The listing builds one solid part. Answer for the finished solid, in the listing's coordinates (mm). A direction names the side the tool comes from. Coordinates: 2 decimals unless noted, no trailing zeros. Loops run counter-clockwise (first coordinate to the right, second up) from the corner with the lowest first, then second, coordinate; pieces in that order, holes last. Notation, with made-up numbers: (0, 2) -> (30, 2) arc R22 cw to (30, 11) -> close; hole circle Ø10 at (-6, -1.75). An arc over 180 degrees is marked (long way). Answer in a Markdown table with one row per item.
```python
from build123d import *

# Parameters (mm, degrees)
EXTRUDE_1_DEPTH          = 18
SKETCH_3_R               = 2.75
CUT_EXTRUDE_1_DEPTH      = 1
CUT_EXTRUDE_1_DEPTH_BACK = 41
CUT_EXTRUDE_2_REACH      = 42
SKETCH_4_R               = 2.75


with BuildPart() as part:
    # 草图1 → 凸台-拉伸1 (new body)
    with BuildSketch(Plane(origin=(0, 0, 0), x_dir=(0, 0, -1), z_dir=(1, 0, 0))):
        Polygon((0, 0), (0, -40), (40, -40), (40, -37), (3, -37), (3, 0), align=None)
    extrude(amount=EXTRUDE_1_DEPTH)

    # 草图3 → 切除-拉伸1 (cut, two sides)
    with BuildSketch(Plane.XZ.offset(40)) as cut_extrude_1_sk:
        with Locations((9, -10)):
            Circle(SKETCH_3_R)
        with Locations((9, -30)):
            Circle(SKETCH_3_R)
    extrude(amount=CUT_EXTRUDE_1_DEPTH, mode=Mode.SUBTRACT)
    extrude(cut_extrude_1_sk.sketch, amount=-CUT_EXTRUDE_1_DEPTH_BACK, mode=Mode.SUBTRACT)

    # 草图4 → 切除-拉伸2 (cut, up to next)
    with BuildSketch(Plane(origin=(0, 0, 0), x_dir=(-1, 0, 0), z_dir=(0, 0, 1)), mode=Mode.PRIVATE) as cut_extrude_2_sk1:
        with Locations((-9, 30)):
            Circle(SKETCH_4_R)
    cut_extrude_2_tool1 = extrude(cut_extrude_2_sk1.sketch, amount=-CUT_EXTRUDE_2_REACH, mode=Mode.PRIVATE) & part.part
    add(cut_extrude_2_tool1.solids().sort_by_distance((9, -30, 0))[0], mode=Mode.SUBTRACT)
    # 草图4 → 切除-拉伸2 (cut, up to next)
    with BuildSketch(Plane(origin=(0, 0, 0), x_dir=(-1, 0, 0), z_dir=(0, 0, 1)), mode=Mode.PRIVATE) as cut_extrude_2_sk2:
        with Locations((-9, 10)):
            Circle(SKETCH_4_R)
    cut_extrude_2_tool2 = extrude(cut_extrude_2_sk2.sketch, amount=-CUT_EXTRUDE_2_REACH, mode=Mode.PRIVATE) & part.part
    add(cut_extrude_2_tool2.solids().sort_by_distance((9, -10, 0))[0], mode=Mode.SUBTRACT)


solid = part.part
```
Item 1: A cutting plane is placed at C-C, the plane y = -30. Determine the outline of the cut face in (x, z).
Findings below:
| item | result |
|---|---|
| outline | (0, -3) -> (6.25, -3) -> (6.25, 0) -> (0, 0) -> close; (11.75, -3) -> (18, -3) -> (18, 0) -> (11.75, 0) -> close |
Item 2: A cutting plane is placed at D-D, the plane x = 12.5. Determine the outline of the cut face in (y, z), plus the area to 3 significant figures.
Findings below:
| item | result |
|---|---|
| outline | (-40, -40) -> (-37, -40) -> (-37, -3) -> (0, -3) -> (0, 0) -> (-40, 0) -> close |
| area | 231 mm2 |
Item 3: Find the intervals of material crossed by probe 1 along Y at (x, z) = (9, -0.8); probe 2 along X at (y, z) = (-10, -1), in increasing order.
Findings below:
| item | result |
|---|---|
| probe 1 | y = -40 to -32.75, -27.25 to -12.75, -7.25 to 0 |
| probe 2 | x = 0 to 6.25, 11.75 to 18 |
Item 4: Flat-ended cylindrical pins translate along their axes: pin 1 Ø4.5 at (x, y) = (9, -30) entering from +Z; pin 2 Ø1 at (x, y) = (2, -5) entering from -Z; pin 3 Ø8 at (x, z) = (2, -15.5) entering from +Y. Find the tip coordinate at first contact, or state that the pin passes through.
Findings below:
| item | result |
|---|---|
| pin 1 | passes through |
| pin 2 | stops at z = -3 |
| pin 3 | stops at y = -37 |
Item 5: A cutting plane is placed at A-A, the plane z = -30. Determine the outline of the cut face in (x, y), plus the area to 3 significant figures.
Findings below:
| item | result |
|---|---|
| outline | (0, -40) -> (6.25, -40) -> (6.25, -37) -> (0, -37) -> close; (11.75, -40) -> (18, -40) -> (18, -37) -> (11.75, -37) -> close |
| area | 37.5 mm2 |
Item 6: A tool of negligible diameter and unlimited length cuts with its end or side. For faces 1 (the face through (9, 0, -2)), 2 (the face through (9, -19, -3)), from which of +Z, -Z, +X, -X, +Y, -Y can it reach the whole face along a straight path? Write none if from no direction.
Findings below:
| item | result |
|---|---|
| face 1 | +Z, -Z, +X, -X, +Y |
| face 2 | -Z, +X, -X, +Y |
Item 7: Determine the mould class of faces 3 (the face through (9, -20, 0)), 4 (the face through (7.52, -32.32, -1.48)), 5 (the face through (9, -37, -22)), 6 (the face through (9, -40, -20)) for opening direction Y: +Y half, -Y half, draft (parallel to the pull), parting line (faces both ways), or undercut.
Findings below:
| item | result |
|---|---|
| face 3 | draft |
| face 4 | undercut |
| face 5 | +Y half |
| face 6 | -Y half |
Item 8: A cutting plane is placed at B-B, the plane x = 9. Determine the outline of the cut face in (y, z).
Findings below:
| item | result |
|---|---|
| outline | (-40, -40) -> (-37, -40) -> (-37, -32.75) -> (-40, -32.75) -> close; (-40, -27.25) -> (-37, -27.25) -> (-37, -12.75) -> (-40, -12.75) -> close; (-40, -7.25) -> (-37, -7.25) -> (-37, -3) -> (-32.75, -3) -> (-32.75, 0) -> (-40, 0) -> close; (-27.25, -3) -> (-12.75, -3) -> (-12.75, 0) -> (-27.25, 0) -> close; (-7.25, -3) -> (0, -3) -> (0, 0) -> (-7.25, 0) -> close |
